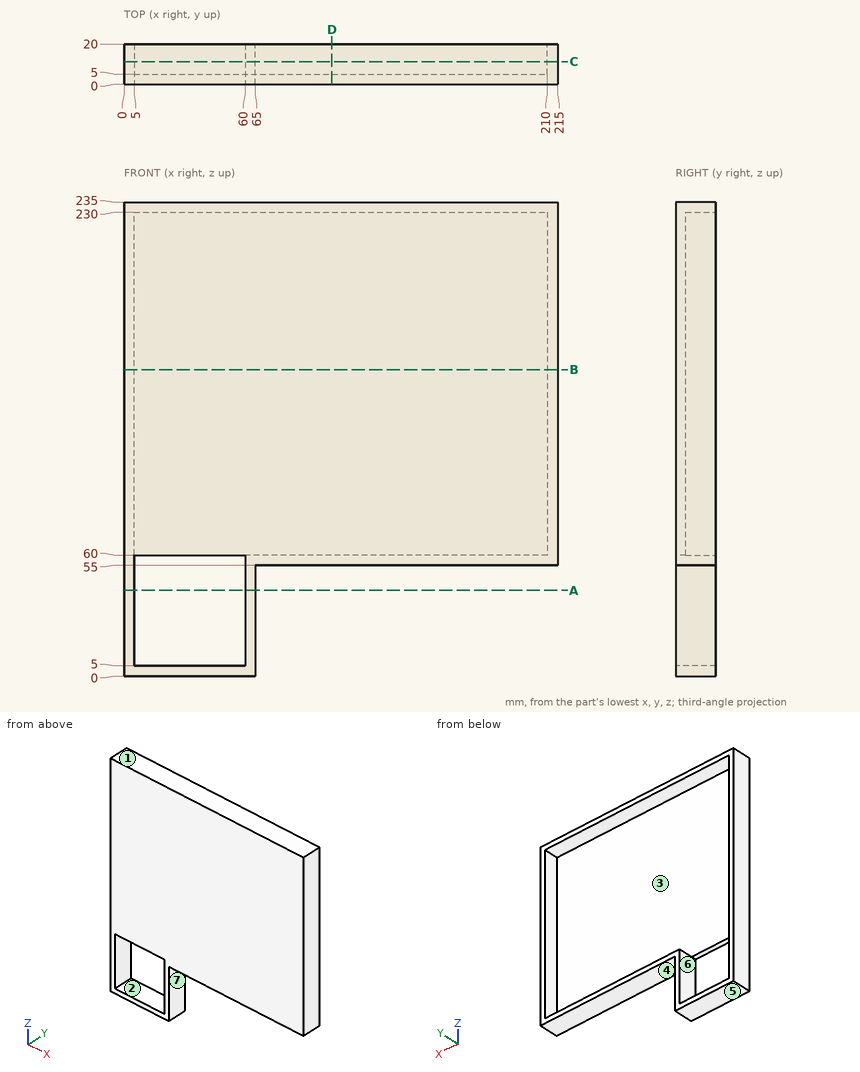
The figure shows three views and two pictorial views of one solid part (mm, origin at its lowest corner). Answer the questions. A direction names the side the tool comes from. Round coordinates to 2 decimals unless told otherwise and drop trailing zeros. Write each loop counter-clockwise with the first axis right and the second up, starting at its lowest first coordinate (ties: lowest second). Pieces come first, ordered by that corner, then holes. Notation, with made-up numbers: (72.25, 35) - (120.25, 35) arc R35 ccw to (120.25, 74) - close; hole circle Ø5 at (37.5, -7). An arc over 180 degrees is marked (long way). Use one line per item in the form item = value. Start each with the question number.
Item 1: A cutting plane is placed at A-A (z = 42.5). Write down the section's boundary in (x, y), plus the area to 3 significant figures.
Item 2: A cutting plane is placed at D-D (x = 103). Write down the section's boundary in (y, z), plus the area to 3 significant figures.
Item 3: Determine the mould class of the marked faces 5, 6 and 7 for opening direction X: +X half, -X half, draft (parallel to the pull), parting line (faces both ways), or undercut.
Item 4: A cutting plane is placed at B-B (z = 152). Write down the section's boundary in (x, y).
Item 5: Find the intervals of material crossed by line 1 (Z direction, x = 126.5, y = 8.25); line 2 (Z direction, x = 34, y = 3.5); line 3 (X direction, y = 14.5, z = 182.5), in increasing order. Write a range as [from, to].
Item 6: Flat-ended cylindrical pins translate along their axes: pin 1 Ø6 at (x, y) = (156, 10) entering from -Z; pin 2 Ø5 at (y, z) = (14, 50.5) entering from +X; pin 3 Ø6 at (x, z) = (103, 209.5) entering from +Y. Find the tip coordinate at first contact, or state that the pin passes through.
Item 7: A cutting plane is placed at C-C (y = 11.25). Write down the section's boundary in (x, z).
Item 8: A tool of negligible diameter and unlimited length cuts with its end or side. For the marked faces 1, 2, 3 and 4, from which of +Z, -Z, +X, -X, +Y, -Y can it reach the whole face along a straight path? Write none if from no direction.
The answers:
q1.outline = (0, 0) - (5, 0) - (5, 20) - (0, 20) - close; (60, 0) - (65, 0) - (65, 20) - (60, 20) - close
q1.area = 200 mm^2
q2.outline = (0, 55) - (20, 55) - (20, 60) - (5, 60) - (5, 230) - (20, 230) - (20, 235) - (0, 235) - close
q2.area = 1,050 mm^2
q3.face_5 = draft
q3.face_6 = undercut
q3.face_7 = +X half
q4.outline = (0, 0) - (215, 0) - (215, 20) - (210, 20) - (210, 5) - (5, 5) - (5, 20) - (0, 20) - close
q5.line_1 = [55, 60], [230, 235]
q5.line_2 = [0, 5], [60, 235]
q5.line_3 = [0, 5], [210, 215]
q6.pin_1 = 55
q6.pin_2 = 65
q6.pin_3 = 5
q7.outline = (0, 0) - (65, 0) - (65, 55) - (215, 55) - (215, 235) - (0, 235) - close; hole (5, 5) - (60, 5) - (60, 60) - (210, 60) - (210, 230) - (5, 230) - close
q8.face_1 = +Z, +X, -X, +Y, -Y
q8.face_2 = +Y, -Y
q8.face_3 = +Y
q8.face_4 = -Z, +X, +Y, -Y
